The drawing under review shows one solid part. Ordinate dimensions are in mm from its lowest x, y, z. A direction names the side the tool comes from. Give positions to 0.01 mm unless a question says otherwise; leave off trailing zeros. Order: outer loops, then holes, each group sorted by start corner. A loop starts at its lowest first (then second) coordinate and runs counter-clockwise, first axis right, second up. Notation, with made-up numbers: (61, 56.5) -> (110, 56.5) arc R21 cw to (110, 77.5) -> close; hole circle Ø10 at (42.5, 16.5). An arc over 180 degrees is marked (long way). Use a Markdown table: item, result. Add a question column.
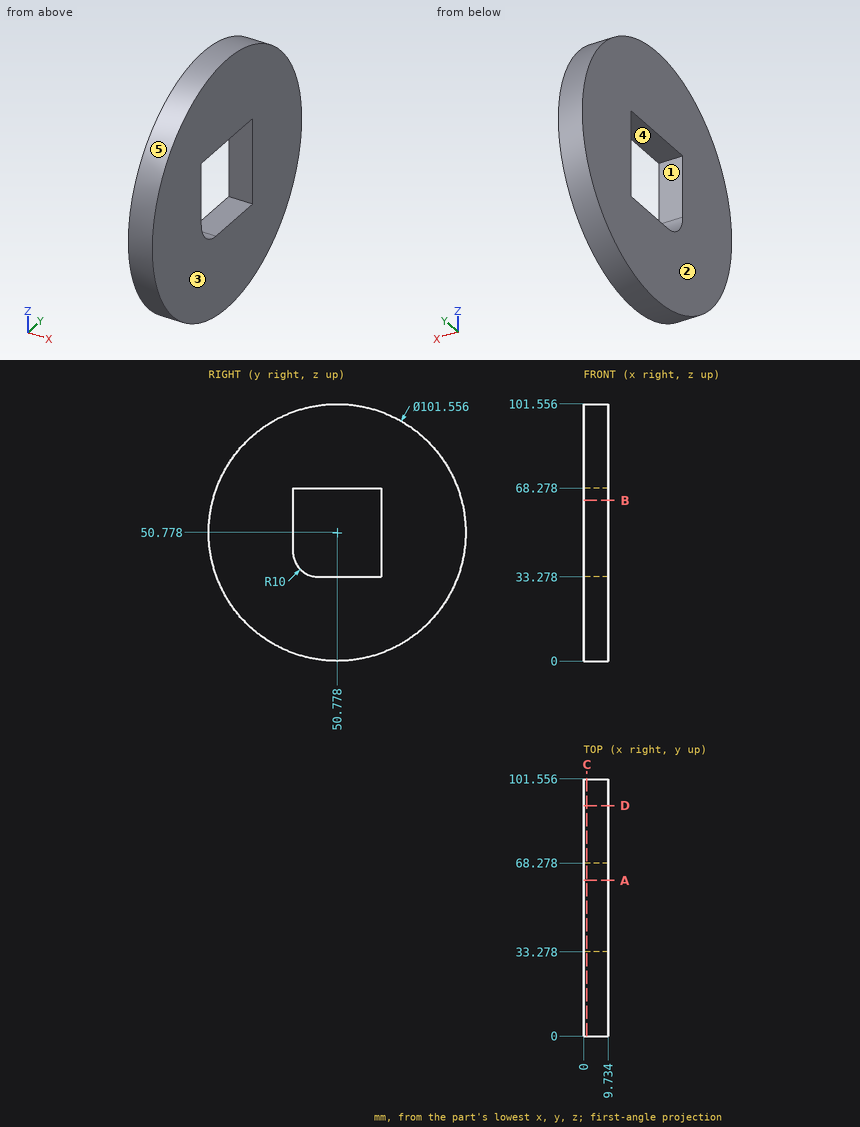
1) Add section A-A (y = 61.5). Give the boundary of the cut face in (x, z) (1 decimal).
2) Machinability: for the marked faces 1 and 2, which of the approach directions +Z, -Z, +X, -X, +Y, -Y give a long, thin tool a straight path to every point of the face, cutting with its end or side? Answer none if there is none.
3) For L1, parallel to Y at x = 6.25, z = 49.5; L2, parallel to Y at x = 6, z = 38 (1 decimal); L3, parallel to Z at x = 6.5, y = 55.5, list the stretches that pass through material, from the lowest coordinate up. Write a range as [from, to].
4) Add section D-D (y = 91). Give the boundary of the cut face in (x, z) (1 decimal), then the cut area to 3 significant figures.
5) The part is to be moulded in two halves that separate along Z. For the marked faces 3, 4 and 5, say which applies: +Z half, -Z half, draft (parallel to the pull), parting line (faces both ways), or undercut.
6) Add section C-C (x = 1.25). Give the boundary of the cut face in (y, z).
7) Insertion check: pin 1 (1 mm diameter, centred on x = 5, z = 58.5, fed in from +Y); pin 2 (1 mm diameter, centred on x = 3.5, z = 33, fed in from -Y); pin 3 (5 mm diameter, centred on x = 3, z = 13, fed in from -Y) (1 decimal). Each pin has a flat end and moves straight along its axis. Give the tip position at first contact, or say it passes through.
8) Add section B-B (z = 63.5). Give the boundary of the cut face in (x, y).
Worked answers:
| question | item | result |
|---|---|---|
| 1 | outline | (0, 1.1) -> (9.7, 1.1) -> (9.7, 33.3) -> (0, 33.3) -> close; (0, 68.3) -> (9.7, 68.3) -> (9.7, 100.4) -> (0, 100.4) -> close |
| 2 | face 1 | +X, -X |
| 2 | face 2 | +Z, -Z, -X, +Y, -Y |
| 3 | L1 | [0.02, 33.28], [68.28, 101.54] |
| 3 | L2 | [1.6, 34.8], [68.3, 99.9] |
| 3 | L3 | [0.22, 33.28], [68.28, 101.34] |
| 4 | outline | (0, 19.8) -> (9.7, 19.8) -> (9.7, 81.8) -> (0, 81.8) -> close |
| 4 | area | 603 mm^2 |
| 5 | face 3 | draft |
| 5 | face 4 | undercut |
| 5 | face 5 | parting line |
| 6 | outline | circle Ø101.56 at (50.78, 50.78); hole (33.28, 43.28) arc R10 ccw to (43.28, 33.28) -> (68.28, 33.28) -> (68.28, 68.28) -> (33.28, 68.28) -> close |
| 7 | pin 1 | y = 101.04 |
| 7 | pin 2 | y = 3.03 |
| 7 | pin 3 | y = 14.3 |
| 8 | outline | (0, 1.62) -> (9.73, 1.62) -> (9.73, 33.28) -> (0, 33.28) -> close; (0, 68.28) -> (9.73, 68.28) -> (9.73, 99.94) -> (0, 99.94) -> close |
